```python
from build123d import *

# Parameters (mm, degrees)
SKETCH1_R      = 3.175
SKETCH1_W      = 25.4
SKETCH1_H      = 6.35
SKETCH1_W_2    = 6.35
SKETCH1_H_2    = 25.4
EXTRUDE2_DEPTH = 6.35
SKETCH2_W      = 6.35
SKETCH2_H      = 25.4
SKETCH2_W_2    = 25.4
SKETCH2_H_2    = 6.35
EXTRUDE4_DEPTH = 399.113447613


with BuildPart() as part:
    # Sketch1 → Extrude2 (new body)
    with BuildSketch(Plane(origin=(0, 0, 0), x_dir=(1, 0, 0), z_dir=(0, 1, 0))):
        with BuildLine():
            Line((-34.925, -292.1), (34.925, -292.1))
            Line((34.925, -292.1), (34.925, -134.703841816))
            ThreePointArc((34.925, -134.703841816), (37.255493422, -127.371493397), (43.391666667, -122.730166988))
            ThreePointArc((43.391666667, -122.730166988), (112.734856938, -65.0875), (127.983275756, 23.786797848))
            ThreePointArc((127.983275756, 23.786797848), (128.934695711, 31.421542964), (134.119449, 37.105983681))
            Line((134.119449, 37.105983681), (270.428520445, 115.804062773))
            Line((270.428520445, 115.804062773), (263.380020445, 128.01242289))
            Line((263.380020445, 128.01242289), (239.953167248, 114.48692289))
            Line((239.953167248, 114.48692289), (243.128167248, 108.987661576))
            Line((243.128167248, 108.987661576), (221.131121992, 96.287661576))
            Line((221.131121992, 96.287661576), (217.956121992, 101.78692289))
            Line((217.956121992, 101.78692289), (206.957599363, 95.43692289))
            Line((206.957599363, 95.43692289), (202.893599363, 102.475977372))
            Line((202.893599363, 102.475977372), (197.394338049, 99.300977372))
            Line((197.394338049, 99.300977372), (184.694338049, 121.298022628))
            Line((184.694338049, 121.298022628), (190.193599363, 124.473022628))
            Line((190.193599363, 124.473022628), (186.129599363, 131.51207711))
            Line((186.129599363, 131.51207711), (197.128121992, 137.86207711))
            Line((197.128121992, 137.86207711), (193.953121992, 143.361338424))
            Line((193.953121992, 143.361338424), (215.950167248, 156.061338424))
            Line((215.950167248, 156.061338424), (219.125167248, 150.56207711))
            Line((219.125167248, 150.56207711), (242.552020445, 164.08757711))
            Line((242.552020445, 164.08757711), (235.503520445, 176.295937227))
            Line((235.503520445, 176.295937227), (99.194449, 97.597858135))
            ThreePointArc((99.194449, 97.597858135), (91.679202289, 95.949950433), (84.591609089, 98.94336914))
            ThreePointArc((84.591609089, 98.94336914), (0, 130.175), (-84.591609089, 98.94336914))
            ThreePointArc((-84.591609089, 98.94336914), (-91.679202289, 95.949950433), (-99.194449, 97.597858135))
            Line((-99.194449, 97.597858135), (-235.503520445, 176.295937227))
            Line((-235.503520445, 176.295937227), (-270.428520445, 115.804062773))
            Line((-270.428520445, 115.804062773), (-134.119449, 37.105983681))
            ThreePointArc((-134.119449, 37.105983681), (-128.934695711, 31.421542964), (-127.983275756, 23.786797848))
            ThreePointArc((-127.983275756, 23.786797848), (-112.734856938, -65.0875), (-43.391666667, -122.730166988))
            ThreePointArc((-43.391666667, -122.730166988), (-37.255493422, -127.371493397), (-34.925, -134.703841816))
            Line((-34.925, -134.703841816), (-34.925, -292.1))
        make_face()
        with Locations(Location((0, 0, 0), (0, 0, 270))):
            Circle(SKETCH1_R, mode=Mode.SUBTRACT)
        with Locations((0, -223.901)):
            Rectangle(SKETCH1_W, SKETCH1_H, mode=Mode.SUBTRACT)
        with Locations((-24.003, -252.476)):
            Rectangle(SKETCH1_W_2, SKETCH1_H_2, mode=Mode.SUBTRACT)
        with Locations((24.003, -252.476)):
            Rectangle(SKETCH1_W_2, SKETCH1_H_2, mode=Mode.SUBTRACT)
        Polygon((-197.504323276, 99.237477372), (-184.804323276, 121.234522628), (-190.30358459, 124.409522628), (-203.00358459, 102.412477372), align=None, mode=Mode.SUBTRACT)
        Polygon((-194.063107218, 143.297838424), (-197.238107218, 137.79857711), (-219.235152474, 150.49857711), (-216.060152474, 155.997838424), align=None, mode=Mode.SUBTRACT)
        Polygon((-240.063152474, 114.42342289), (-243.238152474, 108.924161576), (-221.241107218, 96.224161576), (-218.066107218, 101.72342289), align=None, mode=Mode.SUBTRACT)
    extrude(amount=EXTRUDE2_DEPTH)

    # Sketch2 → Extrude4 (cut, through all)
    with BuildSketch(Plane(origin=(0, 6.35, 0), x_dir=(1, 0, 0), z_dir=(0, 1, 0))):
        with Locations((-31.75, 0)):
            Rectangle(SKETCH2_W, SKETCH2_H)
        with Locations((0, 31.75)):
            Rectangle(SKETCH2_W_2, SKETCH2_H_2)
        with Locations((31.75, 0)):
            Rectangle(SKETCH2_W, SKETCH2_H)
    extrude(amount=-EXTRUDE4_DEPTH, mode=Mode.SUBTRACT)


solid = part.part
```
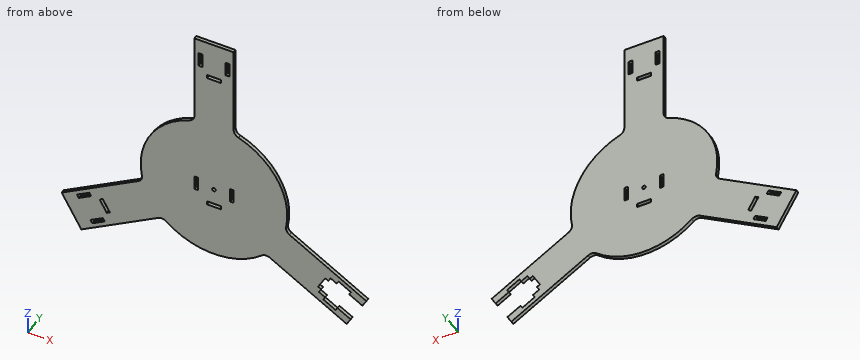
Work out the finished part from the listing and answer in its coordinate system (mm). Give positions to 0.01 mm unless a question says otherwise; leave off trailing zeros. Write each loop counter-clockwise with the first axis right and the second up, starting at its lowest first coordinate (ties: lowest second). Pieces come first, ordered by that corner, then holes. Notation, with made-up numbers: (65, 32) - (122, 32) arc R22 cw to (122, 65) - close; hole circle Ø7 at (21.5, 2). An arc over 180 degrees is marked (long way). Use one line per item in the form item = value.
1. A cutting plane is placed at C-C (y = 1.25). State how many separate pieces and enclosed holes the cut face has, and give its area (3 significant figures).
Filled in:
separate_pieces = 1
enclosed_holes = 10
area = 82,900 mm^2
2. Consider L1, parallel to X at y = 2, z = 0 (3 decimals); L2, parallel to X at y = 2.5, z = -115.5; L3, parallel to Z at x = -232, y = 1.5. Determine where each line is inside the solid, lowest interval first.
Filled in:
L1 = -130.175 to -34.925, -28.575 to -3.175, 3.175 to 28.575, 34.925 to 130.175
L2 = -269.9 to -195.45, -188.12 to -130.2, -60.04 to 60.04, 130.2 to 188.04, 241.71 to 269.9
L3 = -174.27 to -109.77, -102.44 to -93.62
3. Each of these flat-tipped pins is pushed along its axis until it touches: pin 1 Ø1 at (y, z) = (3.5, 59.5) entering from +X; pin 2 Ø3 at (y, z) = (4, -2.5) entering from +X; pin 3 Ø1.9 at (y, z) = (3.5, 3.5) entering from -X; pin 4 Ø4 at (x, z) = (0, 0) entering from -Y. Where does it stop, or does it pass through?
Filled in:
pin_1 = 116.04
pin_2 = 130.17
pin_3 = -130.15
pin_4 = through
4. A cutting plane is placed at A-A (z = 34). Write down the section's boundary in (x, y), and give its area (3 significant figures).
Filled in:
outline = (-125.66, 0) - (125.66, 0) - (125.66, 6.35) - (-125.66, 6.35) - close
area = 1,600 mm^2
5. A cutting plane is placed at B-B (x = 72.5). Write down the section's boundary in (y, z), and give its area (3 significant figures).
Filled in:
outline = (0, -108.12) - (6.35, -108.12) - (6.35, 108.12) - (0, 108.12) - close
area = 1,370 mm^2
